```python
from build123d import *

# Parameters (mm, degrees)
F1_DEPTH    = 25.4
F2_T1_DEPTH = 53.4024208572
F3_DEPTH    = 10.16
F4_DEPTH    = 2.54
F5_W        = 25.4
F5_H        = 3.048
F6_DEPTH    = 7.62
F8_DEPTH    = 5.08


# Not quite as in the source:
# - a fillet or chamfer that OpenCascade refuses, or shapes differently, is made with other operations: its cross-section is extruded or revolved along the edge and cut away or added


with BuildPart() as f1:
    # F0 (on Top) → F1 (new body)
    with BuildSketch(Plane.XY):
        with BuildLine():
            Line((-3.81, -12.7), (3.81, -12.7))
            Line((3.81, -12.7), (3.81, 12.7))
            Line((3.81, 12.7), (-3.81, 12.7))
            Line((-3.81, 12.7), (-3.81, 7.0995158286))
            ThreePointArc((-3.81, 7.0995158286), (-1.4649043996, 3.8885649667), (-0.635, 0))
            ThreePointArc((-0.635, 0), (-1.4649043996, -3.8885649667), (-3.81, -7.0995158286))
            Line((-3.81, -7.0995158286), (-3.81, -12.7))
        make_face()
    extrude(amount=F1_DEPTH)

    # F2: fillet of radius 22.86 on 2 edges, made by hand

    # F2_s2 → F2_t1 (cut)
    with BuildSketch(Plane.XY.offset(-14.0012104286)):
        with BuildLine():
            ThreePointArc((-3.81, 12.7), (-3.1136000163, 8.3102394823), (-1.5809070588, 4.1382108824))
            ThreePointArc((-1.5809070588, 4.1382108824), (-2.5500206467, 5.7283365162), (-3.81, 7.0995158286))
            Line((-3.81, 7.0995158286), (-3.81, 12.7))
        make_face()
        with BuildLine():
            ThreePointArc((-3.81, -12.7), (-3.1136000163, -8.3102394823), (-1.5809070588, -4.1382108824))
            ThreePointArc((-1.5809070588, -4.1382108824), (-2.5500206467, -5.7283365162), (-3.81, -7.0995158286))
            Line((-3.81, -7.0995158286), (-3.81, -12.7))
        make_face()
    extrude(amount=F2_T1_DEPTH, mode=Mode.SUBTRACT)

    # F3 (add): a face of the model
    f3_faces = [f1.faces().sort_by_distance(p)[0] for p in [
        (0.6414875327, 0, 25.4),
    ]]
    extrude(f3_faces, amount=F3_DEPTH)

    # F4 (add): a face of the model
    f4_faces = [f1.faces().sort_by_distance(p)[0] for p in [
        (0.6414875327, 0, 35.56),
    ]]
    extrude(f4_faces, amount=F4_DEPTH)

    # F5 (on face) → F6 (join)
    with BuildSketch(Plane.YZ.offset(3.81)):
        with Locations((0, 12.827)):
            Rectangle(F5_W, F5_H)
        with Locations((0, 6.604)):
            Rectangle(F5_W, F5_H)
    extrude(amount=F6_DEPTH)

    # F7 (on face) → F8 (join)
    with BuildSketch(Plane.XY.offset(8.128)):
        with BuildLine():
            ThreePointArc((3.81, -4.572), (6.427457728, -1.435728864), (7.366, 2.54))
            ThreePointArc((7.366, 2.54), (6.427457728, 6.515728864), (3.81, 9.652))
            Line((3.81, 9.652), (3.81, -4.572))
        make_face()
    extrude(amount=F8_DEPTH)


solid = f1.part
```
Here's how the part is built. I have some questions about the finished solid (model axes, mm). A direction names the side the tool comes from. Round coordinates to 2 decimals unless told otherwise and drop trailing zeros. Loops run counter-clockwise (first coordinate to the right, second up) from the corner with the lowest first, then second, coordinate; pieces in that order, holes last. Notation, with made-up numbers: (72.25, 7.25) -> (76.25, 7.25) arc R20 ccw to (76.25, 30.25) -> close; hole circle Ø6 at (39.25, 89.5). An arc over 180 degrees is marked (long way). Answer as CSV lines item,"result".
1. Which directions (+Z, -Z, +X, -X, +Y, -Y) give clear straight access to the entire face, cutting with the end or side of a thin tool? Please do faces 1 (the face through (3.81, 11, 10)), 2 (the face through (8, 0, 14.351)), 3 (the face through (-3.098, 8.25, 18.783)), 4 (the face through (3.81, -9, 10)), 5 (the face through (8, 0, 5.08)).
Final values:
face 1,"+X, +Y"
face 2,"+Z, +X, +Y, -Y"
face 3,"+Z, -Z, -X"
face 4,"+X, -Y"
face 5,"-Z, +X, +Y, -Y"
2. If we section it at B-B on z = 33.5: Please give me the cut outline in (x, y) (3 decimals), plus the area to 3 significant figures.
Final values:
outline,"(-3.81, -12.7) -> (3.81, -12.7) -> (3.81, 12.7) -> (-3.81, 12.7) arc R22.86 ccw to (-1.581, 4.138) arc R9.525 cw to (-1.581, -4.138) arc R22.86 ccw to start"
area,"156 mm^2"
3. If I drill on L1, parallel to Z at x = 10, y = 1.25; L2, parallel to Z at x = 5, y = 0; L3, parallel to X at y = -9.5, z = 17, over which ranges is the centre line in solid material (lowest first)?
Final values:
L1,"z = 5.08 to 8.13, 11.3 to 14.35"
L2,"z = 5.08 to 14.35"
L3,"x = -3.39 to 3.81"
4. For pin 1 (2 mm diameter, centred on x = 6, y = 10, fed in from -Z); pin 2 (8 mm diameter, centred on y = -2, z = 25.5, fed in from +X); pin 3 (2.5 mm diameter, centred on x = 8.5, y = 2.5, fed in from +Z), each with a flat end and sliding along its axis, tell me the tip position at first contact or that it passes through.
Final values:
pin 1,"stops at z = 5.08"
pin 2,"stops at x = 3.81"
pin 3,"stops at z = 14.35"
5. Thinking about a two-plate mould opening in Y: for faces 6 (the face through (1, 12.7, 19)), 7 (the face through (8, 0, 8.128)), 8 (the face through (-3.13, -8.37, 18.78)), which applies, released by +Y, released by -Y, zero draft, split by the parting line, or undercut?
Final values:
face 6,"released by +Y"
face 7,"zero draft"
face 8,"undercut"
6. If we section it at C-C on y = 6: Please give me the cut outline in (x, z), plus the area to 3 significant figures.
Final values:
outline,"(-2.38, 0) -> (3.81, 0) -> (3.81, 5.08) -> (11.43, 5.08) -> (11.43, 8.13) -> (6.67, 8.13) -> (6.67, 11.3) -> (11.43, 11.3) -> (11.43, 14.35) -> (3.81, 14.35) -> (3.81, 38.1) -> (-2.38, 38.1) -> close"
area,"291 mm^2"
7. If we section it at A-A on x = 9.75: Please give me the cut outline in (y, z), plus the area to 3 significant figures.
Final values:
outline,"(-12.7, 5.08) -> (12.7, 5.08) -> (12.7, 8.13) -> (-12.7, 8.13) -> close; (-12.7, 11.3) -> (12.7, 11.3) -> (12.7, 14.35) -> (-12.7, 14.35) -> close"
area,"155 mm^2"
8. If we section it at D-D on x = -3: Please give me the cut outline in (y, z), plus the area to 3 significant figures.
Final values:
outline,"(-12.7, 0) -> (-7.89, 0) -> (-7.89, 38.1) -> (-12.7, 38.1) -> close; (7.89, 0) -> (12.7, 0) -> (12.7, 38.1) -> (7.89, 38.1) -> close"
area,"366 mm^2"
